from build123d import *

# Parameters (mm, degrees)
F0_W     = 114.3
F0_H     = 38.1
F0_W_2   = 88.9
F0_H_2   = 12.7
F1_DEPTH = 63.5
F2_DEPTH = 12.7
F3_W     = 6.35
F3_H     = 35.56
F4_DEPTH = 15.24
F5_W     = 11.176
F5_H     = 6.35
F6_DEPTH = 12.701
F7_W     = 11.176
F7_H     = 10.16
F8_DEPTH = 18.288
F9_R     = 12.7


with BuildPart() as f1:
    # F0 (on Top) → F1 (new body)
    with BuildSketch(Plane.XY):
        with Locations((57.15, -19.05)):
            Rectangle(F0_W, F0_H)
        with Locations((57.15, -19.05)):
            Rectangle(F0_W_2, F0_H_2, mode=Mode.SUBTRACT)
    extrude(amount=F1_DEPTH)

    # F0 (on Top) → F2 (join)
    with BuildSketch(Plane.XY):
        with Locations((57.15, -19.05)):
            Rectangle(F0_W_2, F0_H_2)
    extrude(amount=F2_DEPTH)

    # F3 (on face) → F4 (cut)
    with BuildSketch(Plane.XZ.offset(38.1)):
        with Locations((17.145, 43.18)):
            Rectangle(F3_W, F3_H)
        with Locations((26.035, 43.18)):
            Rectangle(F3_W, F3_H)
        with Locations((34.925, 43.18)):
            Rectangle(F3_W, F3_H)
        with Locations((43.815, 43.18)):
            Rectangle(F3_W, F3_H)
        with Locations((52.705, 43.18)):
            Rectangle(F3_W, F3_H)
        with Locations((61.595, 43.18)):
            Rectangle(F3_W, F3_H)
        with Locations((70.485, 43.18)):
            Rectangle(F3_W, F3_H)
        with Locations((79.375, 43.18)):
            Rectangle(F3_W, F3_H)
        with Locations((88.265, 43.18)):
            Rectangle(F3_W, F3_H)
        with Locations((97.155, 43.18)):
            Rectangle(F3_W, F3_H)
    extrude(amount=-F4_DEPTH, mode=Mode.SUBTRACT)

    # F5 (on face) → F6 (cut, through all)
    with BuildSketch(Plane.XY.offset(12.7)):
        with Locations((57.15, -19.05)):
            Rectangle(F5_W, F5_H)
    extrude(amount=-F6_DEPTH, mode=Mode.SUBTRACT)

    # F7 (on face) → F8 (cut)
    with BuildSketch(Plane(origin=(0, 0, 0), x_dir=(-1, 0, 0), z_dir=(0, 1, 0))):
        with Locations((-57.15, 5.08)):
            Rectangle(F7_W, F7_H)
    extrude(amount=-F8_DEPTH, mode=Mode.SUBTRACT)

    # F9
    f9_edges = [f1.edges().sort_by_distance(p)[0] for p in [
        (0, -38.1, 31.75),
        (0, 0, 31.75),
        (114.3, -38.1, 31.75),
        (114.3, 0, 31.75),
    ]]
    fillet(f9_edges, radius=F9_R)


solid = f1.part
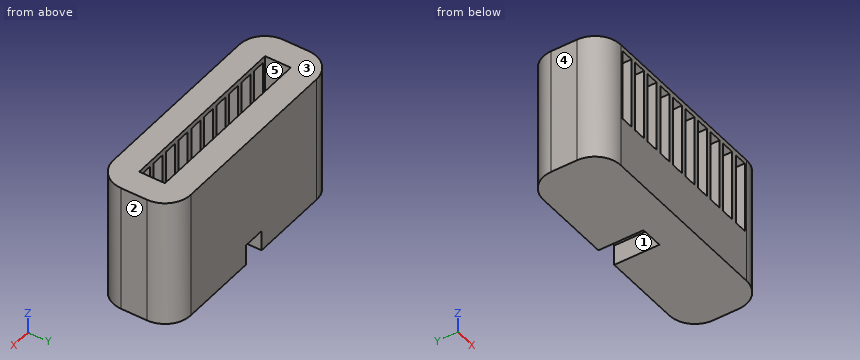
CAD build for the part. Positions are in the model's coordinates, mm. Face numbers are marked on the shaded views. A direction names the side the tool comes from. Give positions to 0.01 mm unless a question says otherwise; leave off trailing zeros. Loops run counter-clockwise (first coordinate to the right, second up) from the corner with the lowest first, then second, coordinate; pieces in that order, holes last. Notation, with made-up numbers: M 74.5,87 L 88.5,87 A10 cw 88.5,93 Z; hole C -8.75,85 d8. An arc over 180 degrees is marked long. Answer in a Markdown table with one row per item. Add a question column.
Item 1: Band-saw the part on C-C on z = 29.5. Give the number of separate pieces and of enclosed holes in the cut face, then the cut area to 3 significant figures.
Item 2: Tool access for the marked faces 4 and 5: list every direction of +Z, -Z, +X, -X, +Y, -Y with a clear straight run to the whole face (end or side of a thin tool).
Item 3: Drop flat-ended pins along their axis: P1, Ø4, axis at x = 43, z = 42.5, coming from the -Y side; P2, Ø6.5, axis at y = -31.5, z = 44, coming from the +X side; P3, Ø4, axis at y = -31.5, z = 36.5, coming from the +X side. Give the stop position or say it passes through.
Item 4: Band-saw the part on B-B on x = 79.5. Give the cut face in (y, z), then the cut area to 3 significant figures.
Item 5: Band-saw the part on D-D on x = 30.5. Give the cut face in (y, z).
Item 6: Probe probe 1 along Y at (x, z) = (31.5, 46); probe 2 along X at (y, z) = (-13, 59.5); probe 3 along Z at (x, y) = (14.5, -29.5). List the from-to ranges inside material, lowest first.
Item 7: Mould opens along X. For the marked faces 1, 2 and 3 say: +X half, -X half, draft (parallel to the pull), parting line (faces both ways), or undercut.
Item 8: Band-saw the part on A-A on x = 53.5. Give the cut face in (y, z) (3 decimals), then the cut area to 3 significant figures.
Reply:
| question | item | result |
|---|---|---|
| 1 | separate pieces | 10 |
| 1 | enclosed holes | 0 |
| 1 | area | 2,280 mm^2 |
| 2 | face 4 | +Z, -Z, -X, +Y, -Y |
| 2 | face 5 | +Z |
| 3 | P1 | stops at y = -12.7 |
| 3 | P2 | stops at x = 113.98 |
| 3 | P3 | stops at x = 113.62 |
| 4 | outline | M -38.1,0 L 0,0 L 0,63.5 L -12.7,63.5 L -12.7,12.7 L -25.4,12.7 L -25.4,25.4 L -38.1,25.4 Z; M -38.1,60.96 L -25.4,60.96 L -25.4,63.5 L -38.1,63.5 Z |
| 4 | area | 1,320 mm^2 |
| 5 | outline | M -38.1,0 L 0,0 L 0,63.5 L -12.7,63.5 L -12.7,12.7 L -25.4,12.7 L -25.4,63.5 L -38.1,63.5 Z |
| 6 | probe 1 | y = -38.1 to -25.4, -12.7 to 0 |
| 6 | probe 2 | x = 0 to 12.7, 101.6 to 114.3 |
| 6 | probe 3 | z = 0 to 25.4, 60.96 to 63.5 |
| 7 | face 1 | undercut |
| 7 | face 2 | +X half |
| 7 | face 3 | draft |
| 8 | outline | M -38.1,0 L -22.225,0 L -22.225,12.7 L -25.4,12.7 L -25.4,25.4 L -38.1,25.4 Z; M -38.1,60.96 L -25.4,60.96 L -25.4,63.5 L -38.1,63.5 Z; M -15.875,10.16 L 0,10.16 L 0,63.5 L -12.7,63.5 L -12.7,12.7 L -15.875,12.7 Z |
| 8 | area | 1,080 mm^2 |
